Part model, mm, in its own coordinate system. A direction names the side the tool comes from. Round coordinates to 2 decimals unless told otherwise and drop trailing zeros. Write each loop counter-clockwise with the first axis right and the second up, starting at its lowest first coordinate (ties: lowest second). Pieces come first, ordered by that corner, then holes. Notation, with made-up numbers: M -33,87.5 L -13,87.5 A19 ccw -13,117.5 Z; hole C 37.25,-40 d2. An arc over 180 degrees is marked long. Answer as a JSON object with one key per item and string values. Group by question number.
1. Band-saw the part on C-C, the plane x = -8.5. Write the cut outline in (y, z), plus the area to 3 significant figures.
2. Which spindle directions (+Z, -Z, +X, -X, +Y, -Y) get a long thin tool onto all of the face, cutting with end or side? Do faces 4 (the face through (-50, -1, 25.4)), 5 (the face through (0, -1, 75)). Say none if no direction does.
3. Band-saw the part on A-A, the plane z = 114.3. Write the cut outline in (x, y).
4. Drill centre lines: line 1 (Z direction, x = -17.5, y = 0); line 2 (X direction, y = -42, z = 120); line 3 (Z direction, x = -36.5, y = 45.5). Where is each one in solid material? Low to high. Write a range as from..to.
5. Band-saw the part on B-B, the plane y = 0. Write the cut outline in (x, z).
6. Two-plate mould, pull along Y, no slides. Class faces 1 (the face through (-12.52, -2.75, 101.9)), 2 (the face through (-22, -76.2, 60)), 3 (the face through (-39, -1, 0)): +Y half, -Y half, draft (parallel to the pull), parting line (faces both ways), or undercut.
7. Drop flat-ended pins along their axis: pin 1 (8 mm diameter, centred on y = 17, z = 107.5, fed in from -X); pin 2 (12 mm diameter, centred on x = -36.5, y = -40, fed in from +Z); pin 3 (12 mm diameter, centred on x = -35.5, z = 39, fed in from -Y). Give the stop position or say it passes through.
8. Band-saw the part on D-D, the plane y = -44. Write the cut outline in (x, z), plus the area to 3 significant figures.
from build123d import *

# Parameters (mm, degrees)
F1_DEPTH = 76.2
F2_R     = 12.7
F3_DEPTH = 76.201


with BuildPart() as f1:
    # F0 (on Front) → F1 (new body, symmetric)
    with BuildSketch(Plane.XZ):
        Polygon((-76.2, 0), (0, 0), (0, 152.4), (-25.4, 152.4), (-25.4, 25.4), (-76.2, 25.4), align=None)
    extrude(amount=F1_DEPTH, both=True)

    # F2 (on face) → F3 (cut, through all)
    with BuildSketch(Plane.YZ):
        with Locations((0, 114.3)):
            Circle(F2_R)
    extrude(amount=-F3_DEPTH, mode=Mode.SUBTRACT)


solid = f1.part
Worked answers:
{
 "1": {"outline": "M -76.2,0 L 76.2,0 L 76.2,152.4 L -76.2,152.4 Z; hole C 0,114.3 d25.4", "area": "22,700 mm^2"},
 "2": {"face 4": "+Z, -X, +Y, -Y", "face 5": "+Z, -Z, +X, +Y, -Y"},
 "3": {"outline": "M -25.4,-76.2 L 0,-76.2 L 0,-12.7 L -25.4,-12.7 Z; M -25.4,12.7 L 0,12.7 L 0,76.2 L -25.4,76.2 Z"},
 "4": {"line 1": "z = 0..101.6, 127..152.4", "line 2": "x = -25.4..0", "line 3": "z = 0..25.4"},
 "5": {"outline": "M -76.2,0 L 0,0 L 0,101.6 L -25.4,101.6 L -25.4,25.4 L -76.2,25.4 Z; M -25.4,127 L 0,127 L 0,152.4 L -25.4,152.4 Z"},
 "6": {"face 1": "undercut", "face 2": "-Y half", "face 3": "draft"},
 "7": {"pin 1": "stops at x = -25.4", "pin 2": "stops at z = 25.4", "pin 3": "passes through"},
 "8": {"outline": "M -76.2,0 L 0,0 L 0,152.4 L -25.4,152.4 L -25.4,25.4 L -76.2,25.4 Z", "area": "5,160 mm^2"}
}
